Answer from the drawing. Dimensions are ordinates in mm from the lowest x, y and z of the part. A direction names the side the tool comes from. Coordinates: 2 decimals unless noted, no trailing zeros. Loops run counter-clockwise (first coordinate to the right, second up) from the corner with the lowest first, then second, coordinate; pieces in that order, holes last. Notation, with made-up numbers: M 78.25,4.5 L 110.25,4.5 A25 ccw 110.25,40.5 Z; hole C 57,-25 d4. An arc over 180 degrees is marked long. Answer as CSV lines item,"result". Start each with the question number.
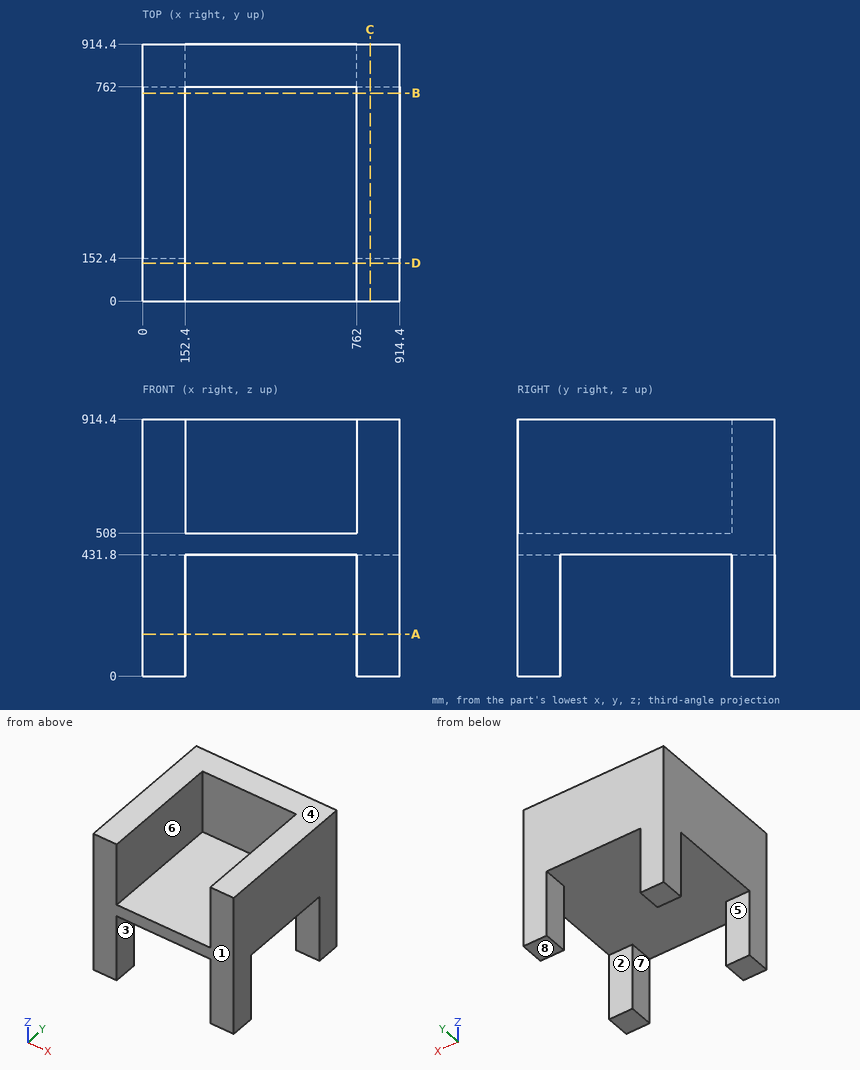
Item 1: For the marked faces 4, 5, 6, 7 and 8, determine the directions among +Z, -Z, +X, -X, +Y, -Y from which every point of the face is accessible in a straight line to the end or side of a thin tool.
Item 2: For a pull along Y with two mould halves and no side action, classify the marked faces 1, 2 and 3 as pulls with the +Y half, pulls with the -Y half, needs draft (parallel to the pull), parting line crosses it, or undercut.
Item 3: Consider line 1 (X direction, y = 349, z = 685.5); line 2 (Z direction, x = 67, y = 164); line 3 (Z direction, x = 611.5, y = 658). Determine where each line is inside the solid, lowest interval first.
Item 4: Section B-B on y = 740 is taken. Determine the outline of the cut face in (x, z).
Item 5: Section D-D on y = 134.5 is taken. Determine the outline of the cut face in (x, z).
Item 6: Each of these flat-tipped pins is pushed along its axis until it touches: P1, Ø2, axis at x = 584, z = 783, coming from the -Y side; P2, Ø2, axis at x = 676, y = 298.5, coming from the +Z side; P3, Ø3, axis at x = 718.5, y = 549, coming from the -Z side. Where does it stop, or does it pass through?
Item 7: Section A-A on z = 149 is taken. Determine the outline of the cut face in (x, y).
Item 8: Section C-C on x = 809.5 is taken. Determine the outline of the cut face in (y, z), then the cut area to 3 significant figures.
Results are:
1,face 4,"+Z, +X, -X, +Y, -Y"
1,face 5,"-Z, +X, -X"
1,face 6,"+Z, -Y"
1,face 7,"-Z, +Y, -Y"
1,face 8,"-Z, +X, -X, +Y, -Y"
2,face 1,"pulls with the -Y half"
2,face 2,"undercut"
2,face 3,"needs draft"
3,line 1,"0 to 152.4, 762 to 914.4"
3,line 2,"431.8 to 914.4"
3,line 3,"431.8 to 508"
4,outline,"M 0,431.8 L 914.4,431.8 L 914.4,914.4 L 762,914.4 L 762,508 L 152.4,508 L 152.4,914.4 L 0,914.4 Z"
5,outline,"M 0,0 L 152.4,0 L 152.4,431.8 L 762,431.8 L 762,0 L 914.4,0 L 914.4,914.4 L 762,914.4 L 762,508 L 152.4,508 L 152.4,914.4 L 0,914.4 Z"
6,P1,"y = 762"
6,P2,"z = 508"
6,P3,"z = 431.8"
7,outline,"M 0,0 L 152.4,0 L 152.4,152.4 L 0,152.4 Z; M 0,762 L 152.4,762 L 152.4,914.4 L 0,914.4 Z; M 762,0 L 914.4,0 L 914.4,152.4 L 762,152.4 Z; M 762,762 L 914.4,762 L 914.4,914.4 L 762,914.4 Z"
8,outline,"M 0,0 L 152.4,0 L 152.4,431.8 L 762,431.8 L 762,0 L 914.4,0 L 914.4,914.4 L 0,914.4 Z"
8,area,"573,000 mm²"
